```python
from build123d import *

# Parameters (mm, degrees)
F0_R        = 15.75
F0_R_2      = 11.25
F1_DEPTH    = 5
F2_R        = 22.5
F2_R_2      = 11.25
F3_DEPTH    = 3
F4_R        = 11.25
F4_R_2      = 10.25
F5_DEPTH    = 1
F6_S5_R     = 11.25
F6_T6_DEPTH = 17
F7_R        = 1


# Not quite as in the source:
# - a fillet or chamfer that OpenCascade refuses, or shapes differently, is made with other operations: its cross-section is extruded or revolved along the edge and cut away or added


with BuildPart() as f1:
    # F0 (on Top) → F1 (new body)
    with BuildSketch(Plane.XY):
        Circle(F0_R)
        Circle(F0_R_2, mode=Mode.SUBTRACT)
    extrude(amount=F1_DEPTH)

    # F2 (on face) → F3 (join)
    with BuildSketch(Plane(origin=(0, 0, 0), x_dir=(1, 0, 0), z_dir=(0, 0, -1))):
        Circle(F2_R)
        Circle(F2_R_2, mode=Mode.SUBTRACT)
    extrude(amount=F3_DEPTH)

    # F4 (on face) → F5 (join)
    with BuildSketch(Plane.XY.offset(5)):
        Circle(F4_R)
        Circle(F4_R_2, mode=Mode.SUBTRACT)
    extrude(amount=-F5_DEPTH)

    # F6: chamfer of 1 x 1.7320508076 on 1 edges, made by hand


with BuildPart() as f6_tool2:
    # F6_s3 → F6_t4 (revolve)
    with BuildSketch(Plane.XZ):
        Polygon((10.25, 5.7320508076), (11.25, 4), (10.25, 4), align=None)
    revolve(axis=Axis((0, 0, 4), (0, 0, 1)))

    # F6_s5 → F6_t6 (intersect, symmetric)
    with BuildSketch(Plane.XY.offset(4.9)):
        Circle(F6_S5_R)
    extrude(amount=F6_T6_DEPTH, both=True, mode=Mode.INTERSECT)


with BuildPart() as f1_1:
    add(f1.part)

    # F6_t1: cut F6_tool2
    add(f6_tool2.part, mode=Mode.SUBTRACT)

    # F7
    f7_edges = [f1_1.edges().sort_by_distance(p)[0] for p in [
        (-15.75, 0, 5),
    ]]
    fillet(f7_edges, radius=F7_R)


solid = f1_1.part
```
Read the model definition and answer for the solid it produces. Units are mm, in the model's axes. Round coordinates to 2 decimals unless told otherwise and drop trailing zeros. Write each loop counter-clockwise with the first axis right and the second up, starting at its lowest first coordinate (ties: lowest second). Pieces come first, ordered by that corner, then holes. Notation, with made-up numbers: (64.5, 81) - (85.5, 81) arc R17 cw to (85.5, 114) - close; hole circle Ø4 at (17, 75). An arc over 180 degrees is marked (long way). Use CSV: the item, a comma, the result in double quotes.
Q1. Find section A-A, the plane x = 0. Write down the section's boundary in (y, z).
Values:
outline,"(-22.5, -3) - (-11.25, -3) - (-11.25, 4) - (-10.67, 5) - (-14.75, 5) arc R1 ccw to (-15.75, 4) - (-15.75, 0) - (-22.5, 0) - close; (10.67, 5) - (11.25, 4) - (11.25, -3) - (22.5, -3) - (22.5, 0) - (15.75, 0) - (15.75, 4) arc R1 ccw to (14.75, 5) - close"
Q2. Determine the mould class of faces 1 (the flat face through (4.7, -15.3, 0)), 2 (the cylindrical face through (5.19, 9.98, 0.55)), 3 (the cylindrical face through (-2.05, 15.616, 1.972)) for opening direction X: +X half, -X half, draft (parallel to the pull), parting line (faces both ways), or undercut.
Values:
face 1,"draft"
face 2,"undercut"
face 3,"parting line"
Q3. Each of these flat-tipped pins is pushed along its axis until it touches: pin 1 Ø2 at (x, y) = (11.5, 11) entering from +Z; pin 2 Ø2 at (x, z) = (2.5, -1.5) entering from +Y. Where does it stop, or does it pass through?
Values:
pin 1,"stops at z = 4.99"
pin 2,"stops at y = 22.45"
Q4. Find section D-D, the plane z = 3.25. Write down the section's boundary in (x, y).
Values:
outline,"circle Ø31.5 at (0, 0); hole circle Ø22.5 at (0, 0)"
Q5. Straight lines are drawn through the part: line 1 along Y through (x, z) = (0, 1.5); line 2 along X through (y, z) = (0, -1); line 3 along X through (y, z) = (-6, 4.5). For each, find the intervals that lie inside material, in ascending order.
Values:
line 1,"y = -15.75 to -11.25, 11.25 to 15.75"
line 2,"x = -22.5 to -11.25, 11.25 to 22.5"
line 3,"x = -14.42 to -9.17, 9.17 to 14.42"
Q6. Find section B-B, the plane z = -1.5. Write down the section's boundary in (x, y), then the cut area to 3 significant figures.
Values:
outline,"circle Ø45 at (0, 0); hole circle Ø22.5 at (0, 0)"
area,"1,190 mm²"
